```python
from build123d import *

# Parameters (mm, degrees)
SKETCH_1_R      = 1.35
EXTRUDE_3_DEPTH = 13
FILLET_1_R      = 3
CHAMFER_1_SIZE  = 1


with BuildPart() as part:
    # 草图1 → 凸台-拉伸3 (new body)
    with BuildSketch(Plane.XY):
        with BuildLine():
            Line((3, 11.4514), (35, 11.4514))
            Line((35, 11.4514), (67, 11.4514))
            ThreePointArc((67, 11.4514), (72.7257, 5.7257), (67, 0))
            Line((67, 0), (35, 0))
            Line((35, 0), (3, 0))
            ThreePointArc((3, 0), (-2.7257, 5.7257), (3, 11.4514))
        make_face()
        with Locations(Location((35, 5.7257, 0), (0, 0, 180))):
            Circle(SKETCH_1_R, mode=Mode.SUBTRACT)
        with Locations(Location((3, 5.7257, 0), (0, 0, 180))):
            Circle(SKETCH_1_R, mode=Mode.SUBTRACT)
        with Locations(Location((67, 5.7257, 0), (0, 0, 180))):
            Circle(SKETCH_1_R, mode=Mode.SUBTRACT)
        with BuildLine():
            Line((7.071532881, 9.7514), (18.014251374, 9.7514))
            Line((18.014251374, 9.7514), (18.014251374, 1.7))
            Line((18.014251374, 1.7), (7.071532881, 1.7))
            ThreePointArc((7.071532881, 1.7), (8.7257, 5.7257), (7.071532881, 9.7514))
        make_face(mode=Mode.SUBTRACT)
        with BuildLine():
            Line((20.014251374, 9.7514), (20.014251374, 1.7))
            Line((20.014251374, 1.7), (30.928467119, 1.7))
            ThreePointArc((30.928467119, 1.7), (29.2743, 5.7257), (30.928467119, 9.7514))
            Line((30.928467119, 9.7514), (20.014251374, 9.7514))
        make_face(mode=Mode.SUBTRACT)
        with BuildLine():
            Line((39.071532881, 9.7514), (50.013401562, 9.7514))
            Line((50.013401562, 9.7514), (50.013401562, 1.7))
            Line((50.013401562, 1.7), (39.071532881, 1.7))
            ThreePointArc((39.071532881, 1.7), (40.7257, 5.7257), (39.071532881, 9.7514))
        make_face(mode=Mode.SUBTRACT)
        with BuildLine():
            Line((62.928467119, 9.7514), (52.013401562, 9.7514))
            Line((52.013401562, 9.7514), (52.013401562, 1.7))
            Line((52.013401562, 1.7), (62.928467119, 1.7))
            ThreePointArc((62.928467119, 1.7), (61.2743, 5.7257), (62.928467119, 9.7514))
        make_face(mode=Mode.SUBTRACT)
    extrude(amount=EXTRUDE_3_DEPTH)

    # 圆角1
    fillet_1_edges = [part.edges().sort_by_distance(p)[0] for p in [
        (20.014251374, 9.7514, 6.5),
        (20.014251374, 1.7, 6.5),
        (50.013401562, 1.7, 6.5),
        (50.013401562, 9.7514, 6.5),
        (52.013401562, 9.7514, 6.5),
        (52.013401562, 1.7, 6.5),
        (18.014251374, 1.7, 6.5),
        (18.014251374, 9.7514, 6.5),
    ]]
    fillet(fillet_1_edges, radius=FILLET_1_R)

    # 倒角1
    chamfer_1_edges = [part.edges().sort_by_distance(p)[0] for p in [
        (72.7257, 5.7257, 13),
        (35, 11.4514, 13),
        (-2.7257, 5.7257, 13),
        (35, 11.4514, 0),
        (72.7257, 5.7257, 0),
        (35, 0, 0),
        (-2.7257, 5.7257, 0),
        (35, 0, 13),
    ]]
    chamfer(chamfer_1_edges, length=CHAMFER_1_SIZE)


solid = part.part
```
Check sheet for the modelled part. Datum: model origin and axes. Units: mm. A direction names the side the tool comes from. Round coordinates to 2 decimals unless told otherwise and drop trailing zeros. Order: outer loops, then holes, each group sorted by start corner. A loop starts at its lowest first (then second) coordinate and runs counter-clockwise, first axis right, second up. Notation, with made-up numbers: M 82,69 L 116,69 A22 ccw 116,89 Z; hole C -14,67.5 d5. An arc over 180 degrees is marked long. Answer in a Markdown table with one row per item.
(1) Section check A-A on x = 35. Record the boundary of the cut face in (y, z), plus the area to 3 significant figures.
Findings:
| item | result |
|---|---|
| outline | M 0,1 L 1,0 L 4.38,0 L 4.38,13 L 1,13 L 0,12 Z; M 7.08,0 L 10.45,0 L 11.45,1 L 11.45,12 L 10.45,13 L 7.08,13 Z |
| area | 112 mm^2 |
(2) Set-up check for faces 4 (the conical face through (-1.898, 5.618, 12.826)), 5 (the flat face through (43, 9.751, 6)): record each of +Z, -Z, +X, -X, +Y, -Y from which the full face is reachable in a straight line by a thin tool's end or side.
Findings:
| item | result |
|---|---|
| face 4 | +Z, -X |
| face 5 | +Z, -Z |
(3) Section check C-C on x = 12. Record the boundary of the cut face in (y, z).
Findings:
| item | result |
|---|---|
| outline | M 0,1 L 1,0 L 1.7,0 L 1.7,13 L 1,13 L 0,12 Z; M 9.75,0 L 10.45,0 L 11.45,1 L 11.45,12 L 10.45,13 L 9.75,13 Z |
(4) Material ranges on line 1 along Y through (x, z) = (3, 6.75); line 2 along X through (y, z) = (4.25, 1.5); line 3 along X through (y, z) = (3, 12.25), recorded low to high. Write a range as from..to.
Findings:
| item | result |
|---|---|
| line 1 | y = 0..4.38, 7.08..11.45 |
| line 2 | x = -2.53..8.53, 17.98..20.05, 29.47..40.53, 49.98..52.05, 61.47..72.53 |
| line 3 | x = -1.75..8.04, 17.49..20.54, 29.96..40.04, 49.49..52.54, 61.96..71.75 |
(5) Draft check along X on faces 1 (the conical face through (71.898, 5.833, 12.826)), 2 (the flat face through (52.013, 6, 6)), 3 (the conical face through (-1.898, 5.618, 0.174)). Enter one of: +X half, -X half, draft (parallel to the pull), parting line (faces both ways), or undercut.
Findings:
| item | result |
|---|---|
| face 1 | +X half |
| face 2 | undercut |
| face 3 | -X half |
(6) Section check B-B on z = 8. Give the number of separate pieces and of enclosed holes in the cut face, plus the area to 3 significant figures.
Findings:
| item | result |
|---|---|
| separate pieces | 1 |
| enclosed holes | 7 |
| area | 519 mm^2 |
